Input: dimensioned drawing with shaded views. Units: mm. Origin: part minimum x, y, z. A direction names the side the tool comes from. Give positions to 0.01 mm unless a question says otherwise; leave off trailing zeros. Write each loop counter-clockwise with the first axis right and the second up, starting at its lowest first coordinate (ties: lowest second). Pieces come first, ordered by that corner, then holes. Notation, with made-up numbers: (14.25, 57.25) -> (58.25, 57.25) arc R26 ccw to (58.25, 76.25) -> close; hole circle Ø2 at (-8.75, 13). An arc over 180 degrees is marked (long way). Answer as a JSON object with one key per item and string values. Group by question number.
(1) Section query C-C on z = 33. Output: boundary loops of the cut face in (x, y), plus the area to 4 significant figures.
(2) Section query D-D on x = 11. Output: boundary loops of the cut face in (y, z), plus the area to 3 significant figures.
(3) Material intervals for probe 1 along Y at (x, z) = (30, 2); probe 2 along Z at (x, y) = (26, 21) (1 decimal); probe 3 along X at (y, z) = (30, 25) (1 decimal), sorted ascending.
(4) Draft query along Z for the marked faces 3, 4 and 5. Return one class per face: +Z half, -Z half, draft (parallel to the pull), parting line (faces both ways), or undercut.
(5) Section query A-A on x = 34. Output: boundary loops of the cut face in (y, z) (1 decimal).
(6) Section query B-B on y = 26.5. Output: boundary loops of the cut face in (x, z) (1 decimal), plus the area to 3 significant figures.
(7) Set-up query: the marked faces 1 and 2. Return all of +Z, -Z, +X, -X, +Y, -Y with unobstructed straight access to the full face (end or side cutting, diameter ignored); none if empty.
(8) Contact query for flat-ended pins moving along their axis: pin 1 Ø13.5 at (x, z) = (26.13, 20.88) entering from +Y; pin 2 Ø3 at (y, z) = (4, 18) entering from -X; pin 3 Ø10 at (y, z) = (7, 33) entering from -X; pin 4 Ø6 at (y, z) = (8.5, 22.5) entering from +X. Output: stop coordinate, or through.
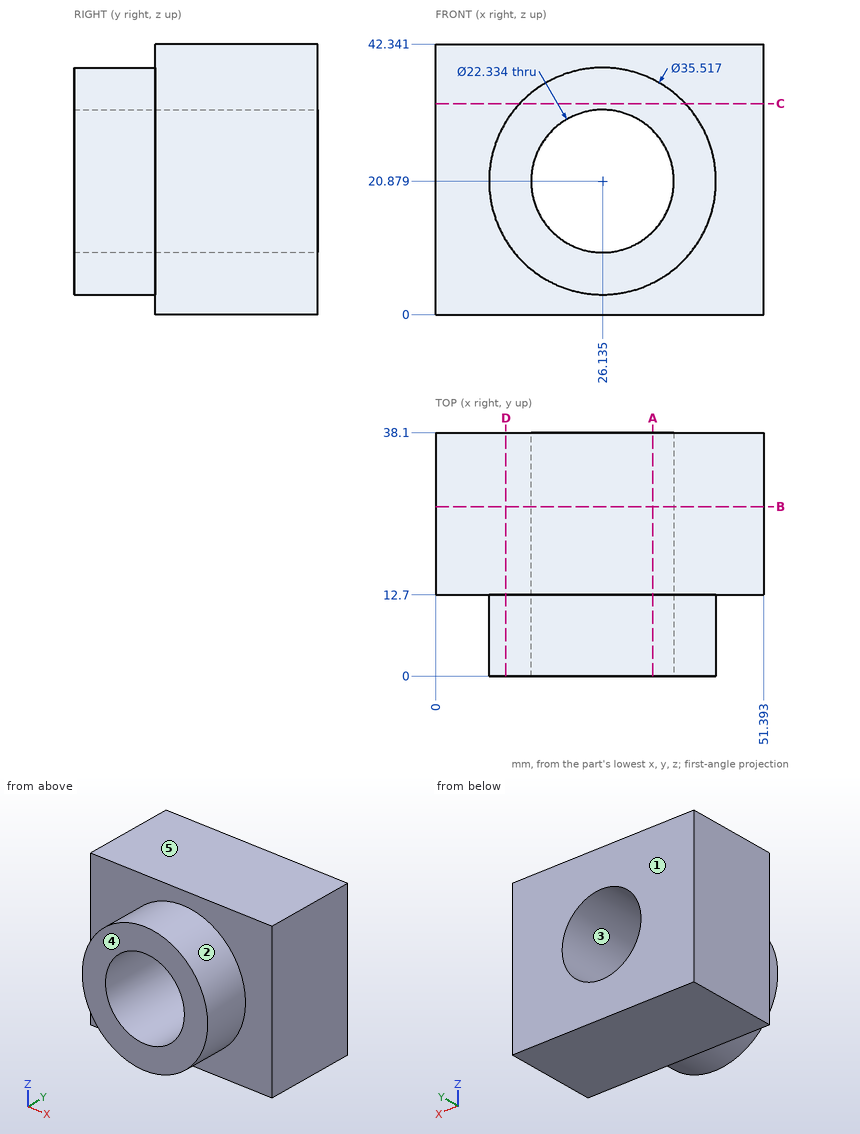
Answer list:
{
 "1": {"outline": "(0, 12.7) -> (13.16, 12.7) -> (13.16, 0) -> (39.11, 0) -> (39.11, 12.7) -> (51.39, 12.7) -> (51.39, 38.1) -> (0, 38.1) -> close", "area": "1,635 mm2"},
 "2": {"outline": "(0, 11.59) -> (12.7, 11.59) -> (12.7, 0) -> (38.1, 0) -> (38.1, 42.34) -> (12.7, 42.34) -> (12.7, 30.17) -> (0, 30.17) -> close", "area": "1,310 mm2"},
 "3": {"probe 1": "12.7 to 38.1", "probe 2": "0 to 9.7, 32 to 42.3", "probe 3": "0 to 15.8, 36.5 to 51.4"},
 "4": {"face 3": "undercut", "face 4": "draft", "face 5": "+Z half"},
 "5": {"outline": "(0, 5) -> (12.7, 5) -> (12.7, 0) -> (38.1, 0) -> (38.1, 13) -> (0, 13) -> close; (0, 28.8) -> (38.1, 28.8) -> (38.1, 42.3) -> (12.7, 42.3) -> (12.7, 36.8) -> (0, 36.8) -> close"},
 "6": {"outline": "(0, 0) -> (51.4, 0) -> (51.4, 42.3) -> (0, 42.3) -> close; hole circle Ø22.3 at (26.1, 20.9)", "area": "1,780 mm2"},
 "7": {"face 1": "+Z, -Z, +X, -X, +Y", "face 2": "-Y"},
 "8": {"pin 1": "through", "pin 2": "x = 8.43", "pin 3": "x = 9.87", "pin 4": "x = 43.89"}
}
